For this review, take the finished solid that the model builds, in its own axes (mm). A direction names the side the tool comes from. Coordinates: 2 decimals unless noted, no trailing zeros. Loops run counter-clockwise (first coordinate to the right, second up) from the corner with the lowest first, then second, coordinate; pieces in that order, holes last. Notation, with made-up numbers: (15, -0.75) -> (36, -0.75) arc R27 cw to (36, 25.25) -> close; hole circle Ø8 at (-24, 64). An arc over 180 degrees is marked (long way). Use a Markdown table: item, result.
Autodesk Inventor part; units mm, degrees
ref_plane "Work Plane1" through (8, 0, 0) normal (0, 0.5, 0.866) x (1, 0, 0)
ref_plane "YZ Plane" through (0, 0, 0) normal (1, 0, 0) x (0, 1, 0)
ref_plane "XZ Plane" through (0, 0, 0) normal (0, 1, 0) x (-1, 0, 0)
sketch "Sketch1" plane through (0, 0, 0) normal (0, 0, 1) x (1, 0, 0)
  line L0 (0, 0) -> (11.5, 0)
  line L1 (16, 1.7321) -> (16, 3)
  line L2 (16, 3) -> (0, 3)
  line L3 (16, 1.7321) -> (12.5, 1.7321)
  line L4 (12.5, 1.7321) -> (11.5, 0)
  line L5 (0, -0.6) -> (0, 3.6)
  line L6 (0, 3) -> (0, 0)
  dimension "d0" = 3.5
  dimension "d1" = 60
  dimension "d2" = 6
  dimension "d3" = 3.4641
  dimension "d5" = 16
revolve "Body" add sketch "Sketch1" angle 360 about axis through (0, 0, 0) along (1, 0, 0)
chamfer "Chamfer1" distance 0.6135 angle 45 1 edges at (16, -3, 0) measured on face at (16, 2.5483, -0.2393)
sketch "Sketch2" plane through (16, 0, 0) normal (1, 0, 0) x (0, 0, -1)
  circle A0 centre (0, 0) radius 1.7321
  line L0 (-0.866, 1.5) -> (0.866, 1.5)
  line L1 (0.866, 1.5) -> (1.7321, 0)
  line L2 (1.7321, 0) -> (0.866, -1.5)
  line L3 (0.866, -1.5) -> (-0.866, -1.5)
  line L4 (-0.866, -1.5) -> (-1.7321, 0)
  line L5 (-1.7321, 0) -> (-0.866, 1.5)
  point P0 (0, 0)
  point P1 (0, 0)
extrude "Slot" add sketch "Sketch2" against normal up to next contours L1 A0 | A0 L2 | L0 A0 | A0 L3 | L5 A0 | A0 L4
thread "Thread"
chamfer "Chamfer2" distance 0.6135 angle 45 1 edges at (0, -3, 0) measured on face at (5.1288, 2.9612, -0.4812)
ref_plane "Work Plane1" through (8, 0, 0) normal (0, 0.5, 0.866) x (1, 0, 0)
equation "\"d7\" = -0.5 * GD1 + 0.5 * NND"
equation "\"d8\" = FAWI"
equation "\"d29\" = -0.5 * GD1 + 0.5 * NND"
equation "\"d11\" = NLG"
equation "\"d13\" = -0.5 * GD1 + 0.5 * NND"
equation "\"d14\" = FAWI"
equation "\"d30\" = -0.5 * GD1 + 0.5 * NND"
equation "\"d0\" = INTI"
equation "\"d2\" = NND"
equation "\"d3\" = 1.1547 * SW"
equation "\"d5\" = NLG"
equation "\"NND\" = 6"
equation "\"NLG\" = 16"
equation "\"INTI\" = 3.5"
equation "\"FAWI\" = 45deg"
equation "\"SW\" = 3"
equation "\"GD1\" = THREADDIA - 1.2269 * PTC"
equation "\"FAWI1\" = 45deg"
equation "\"GUL\" = 0.61345 * PTC"
equation "\"SPD\" = 4"
equation "\"SEWI\" = 90deg"
equation "\"TOA\" = 30deg"
equation "\"THREADDIA\" = 6"
equation "\"PTC\" = 1"
equation "\"GAL\" = 0.61345 * PTC"
equation "\"E0\" = 1.155 * SW"
properties part number "ISO 4026 - M6 x 16" material "Stainless Steel, 440C"
(1) For line 1 along Y through (x, z) = (5.5, 0.1); line 2 along Y through (x, z) = (10, -1.75); line 3 along Z through (x, y) = (7, -1.9), list the stretches that pass through material, from the lowest coordinate up.
Found:
| item | result |
|---|---|
| line 1 | y = -3 to 3 |
| line 2 | y = -2.44 to 2.44 |
| line 3 | z = -2.32 to 2.32 |
(2) Mouldability with a two-part tool opening along Z and no side actions: class faces 1 (the face through (14, -1.5, 0)), 2 (the face through (0, 0, 0)), 3 (the face through (8, -3, 0)) as pulls with the +Z half, pulls with the -Z half, needs draft (parallel to the pull), parting line crosses it, or undercut.
Found:
| item | result |
|---|---|
| face 1 | undercut |
| face 2 | needs draft |
| face 3 | parting line crosses it |
(3) For faces 4 (the face through (16, 2, 0)), 5 (the face through (14.208, -0.74, -1.305)), list the 3-axis set-ups (+Z, -Z, +X, -X, +Y, -Y) from which the entire face can be reached by the end or side of a thin tool; tool diameter is ignored.
Found:
| item | result |
|---|---|
| face 4 | +Z, -Z, +X, +Y, -Y |
| face 5 | +X |
(4) For pin 1 Ø1.5 at (y, z) = (0.5, -0.5) entering from -X; pin 2 Ø2 at (x, y) = (8, -2) entering from -Z; pin 3 Ø1 at (x, z) = (4, 1.5) entering from -Y; pin 4 Ø3 at (x, y) = (9.5, 2) entering from +Z, all flat-tipped, find the tip position at first contact; note any pin that passes through.
Found:
| item | result |
|---|---|
| pin 1 | stops at x = 0 |
| pin 2 | stops at z = -2.83 |
| pin 3 | stops at y = -2.83 |
| pin 4 | stops at z = 2.96 |
(5) Take a section at A-A on x = 5.5. Write out the cut boundary in (y, z).
Found:
| item | result |
|---|---|
| outline | circle Ø6 at (0, 0) |
